Check sheet for the modelled part. Datum: model origin and axes. Units: mm. A direction names the side the tool comes from. Give positions to 0.01 mm unless a question says otherwise; leave off trailing zeros. Order: outer loops, then holes, each group sorted by start corner. A loop starts at its lowest first (then second) coordinate and runs counter-clockwise, first axis right, second up.
```python
from build123d import *

# Parameters (mm, degrees)
SKETCH1_R           = 75
SKETCH1_R_2         = 29
BOSS_EXTRUDE1_DEPTH = 10
SKETCH2_R           = 84.502985649
SKETCH2_R_2         = 57
CUT_EXTRUDE2_DEPTH  = 3
HOLE1_D             = 8.5
HOLE1_CBORE_D       = 12.5
HOLE1_CBORE_DEPTH   = 5
CIRPATTERN1_COUNT   = 4
HOLE2_D             = 7
CIRPATTERN2_COUNT   = 6


with BuildPart() as part:
    # Sketch1 → Boss-Extrude1 (new body)
    with BuildSketch(Plane.XY):
        Circle(SKETCH1_R)
        Circle(SKETCH1_R_2, mode=Mode.SUBTRACT)
    extrude(amount=BOSS_EXTRUDE1_DEPTH)

    # Sketch2 → Cut-Extrude2 (cut)
    with BuildSketch(Plane.XY.offset(10)):
        Circle(SKETCH2_R)
        Circle(SKETCH2_R_2, mode=Mode.SUBTRACT)
    extrude(amount=-CUT_EXTRUDE2_DEPTH, mode=Mode.SUBTRACT)

    # Hole1 (through all)
    with Locations(Plane(origin=(0, 39.25, 10), x_dir=(1, 0, 0), z_dir=(0, 0, 1))):
        with Locations((0, 0)):
            hole1 = CounterBoreHole(HOLE1_D / 2, HOLE1_CBORE_D / 2, HOLE1_CBORE_DEPTH)

    # CirPattern1: Hole1 ×4 about axis
    cirpattern1_axis = Axis((0, 0, 0), (0, 0, 1))
    for i in range(1, CIRPATTERN1_COUNT):
        add(hole1.rotate(cirpattern1_axis, i * 360 / CIRPATTERN1_COUNT), mode=Mode.SUBTRACT)

    # Hole2 (through all)
    with Locations(Plane.XY.offset(7)):
        with Locations((0, 67)):
            hole2 = Hole(HOLE2_D / 2)

    # CirPattern2: Hole2 ×6 about axis
    cirpattern2_axis = Axis((0, 0, 0), (0, 0, 1))
    for i in range(1, CIRPATTERN2_COUNT):
        add(hole2.rotate(cirpattern2_axis, i * 360 / CIRPATTERN2_COUNT), mode=Mode.SUBTRACT)


solid = part.part
```
Q1. Sectioned sample at A-A, the plane y = 0. Record the cut outline in (x, z).
Q2. Tool access check on faces 1 (the cylindrical face through (13.38, -25.73, 4.93)), 2 (the cylindrical face through (45.447, 0.814, 7.535)). Record the directions out of +Z, -Z, +X, -X, +Y, -Y that give a thin tool (end or side, any length) a straight path to the whole face; none if there is none.
Q3. Sectioned sample at B-B, the plane x = -20. Record the cut outline in (y, z), plus the area to 3 significant figures.
Q4. Go/stop test with flat-tipped pins: P1, Ø11, axis at x = 39.25, y = 0, coming from the -Z side; P2, Ø7, axis at x = -39.25, y = 0, coming from the +Z side; P3, Ø4, axis at y = 25.5, z = 5, coming from the +X side; P4, Ø12, axis at x = 51, y = 52.5, coming from the +Z side. Record where each tip stops, or that it passes through.
Q5. Draft check along X on faces 3 (the flat face through (-26.1, 13.5, 10)), 4 (the cylindrical face through (-60.6, 31.13, 3.45)), 5 (the cylindrical face through (52.654, -21.831, 8.521)). Enter one of: pulls with the +X half, pulls with the -X half, needs draft (parallel to the pull), parting line crosses it, or undercut.
Q6. Sectioned sample at C-C, the plane y = -67. Record the cut outline in (x, z), plus the area to 3 significant figures.
Q7. Sectioned sample at D-D, the plane z = 1.5. Count the separate pieces of the cut face and the enclosed holes in it, plus the area to 3 significant figures.
Q8. Material ranges on line 1 (Y direction, x = 0, z = 1.75); line 2 (Y direction, x = -59, z = 6.25); line 3 (Y direction, x = 55, z = 2), recorded low to high.
Filled in:
1. outline: (-75, 0) - (-43.5, 0) - (-43.5, 5) - (-45.5, 5) - (-45.5, 10) - (-57, 10) - (-57, 7) - (-75, 7) - close; (-35, 0) - (-29, 0) - (-29, 10) - (-33, 10) - (-33, 5) - (-35, 5) - close; (29, 0) - (35, 0) - (35, 5) - (33, 5) - (33, 10) - (29, 10) - close; (43.5, 0) - (75, 0) - (75, 7) - (57, 7) - (57, 10) - (45.5, 10) - (45.5, 5) - (43.5, 5) - close
2. face 1: +Z, -Z
2. face 2: +Z
3. outline: (-72.28, 0) - (-21, 0) - (-21, 10) - (-53.38, 10) - (-53.38, 7) - (-72.28, 7) - close; (21, 0) - (72.28, 0) - (72.28, 7) - (53.38, 7) - (53.38, 10) - (21, 10) - close
3. area: 912 mm2
4. P1: stops at z = 0
4. P2: passes through
4. P3: stops at x = 71.22
4. P4: stops at z = 7
5. face 3: needs draft
5. face 4: undercut
5. face 5: parting line crosses it
6. outline: (-33.7, 0) - (-3.5, 0) - (-3.5, 7) - (-33.7, 7) - close; (3.5, 0) - (33.7, 0) - (33.7, 7) - (3.5, 7) - close
6. area: 423 mm2
7. separate pieces: 1
7. enclosed holes: 11
7. area: 14,600 mm2
8. line 1: y = -75 to -70.5, -63.5 to -43.5, -35 to -29, 29 to 35, 43.5 to 63.5, 70.5 to 75
8. line 2: y = -46.3 to -36.86, -30.14 to 30.14, 36.86 to 46.3
8. line 3: y = -50.99 to -35.26, -31.74 to 31.74, 35.26 to 50.99
